from build123d import *

# Parameters (mm, degrees)
SKETCH1_W           = 60
SKETCH1_H           = 5
SKETCH1_W_2         = 50
SKETCH1_H_2         = 10
SKETCH1_W_3         = 5
BOSS_EXTRUDE1_DEPTH = 9
SKETCH1_3_W         = 50
SKETCH1_3_H         = 23
SKETCH1_3_W_2       = 65
SKETCH1_3_H_2       = 90
SKETCH1_3_R         = 1.5
SKETCH1_3_W_3       = 1.5
SKETCH1_3_H_3       = 74
BOSS_EXTRUDE2_DEPTH = 3
SKETCH2_R           = 1.5
BOSS_EXTRUDE3_DEPTH = 3
SKETCH3_R           = 4
CUT_EXTRUDE1_DEPTH  = 5
SKETCH3_3_R         = 1.5
CUT_EXTRUDE2_DEPTH  = 20
SKETCH4_W           = 70
SKETCH4_H           = 9
BOSS_EXTRUDE4_DEPTH = 3
SKETCH3_6_R         = 2.5
SKETCH3_6_R_2       = 1.5
CUT_EXTRUDE5_DEPTH  = 3


with BuildPart() as part:
    # Sketch1 → Boss-Extrude1 (new body)
    with BuildSketch(Plane(origin=(0, 0, 0), x_dir=(1, 0, 0), z_dir=(0, 1, 0))):
        Polygon((-30, -60), (-30, 40), (-30, 45), (-30, 65), (-35, 65), (-35, 25), (-35, -65), (-30, -65), align=None)
        with Locations((0, -62.5)):
            Rectangle(SKETCH1_W, SKETCH1_H)
        Polygon((30, 40), (30, -60), (30, -65), (35, -65), (35, 65), (30, 65), (30, 55), (30, 45), align=None)
        Polygon((-30, 65), (-30, 45), (-25, 45), (-25, 55), (25, 55), (25, 65), align=None)
        with Locations((0, 50)):
            Rectangle(SKETCH1_W_2, SKETCH1_H_2)
        with Locations((27.5, 60)):
            Rectangle(SKETCH1_W_3, SKETCH1_H_2)
        with Locations((27.5, 50)):
            Rectangle(SKETCH1_W_3, SKETCH1_H_2)
    extrude(amount=BOSS_EXTRUDE1_DEPTH)

    # Sketch1_3 → Boss-Extrude2 (add)
    # profile 1 of 2: a face of its own
    with BuildSketch(Plane(origin=(0, 0, 0), x_dir=(1, 0, 0), z_dir=(0, 1, 0))):
        Polygon((-30, 45), (-30, -60), (30, -60), (30, 45), (25, 45), (25, -23), (-25, -23), (-25, 45), align=None)
        with Locations((0, -43.5)):
            Rectangle(SKETCH1_3_W, SKETCH1_3_H, mode=Mode.SUBTRACT)
    # profile 2 of 2: a face of its own
    with BuildSketch(Plane(origin=(0, 0, 0), x_dir=(1, 0, 0), z_dir=(0, 1, 0))):
        with Locations((-67.5, -20)):
            Rectangle(SKETCH1_3_W_2, SKETCH1_3_H_2)
        with Locations(Location((-42.5, 22.5, 0), (0, 0, 270))):
            Circle(SKETCH1_3_R, mode=Mode.SUBTRACT)
        with Locations(Location((-57.5, -62.5, 0), (0, 0, 270))):
            Circle(SKETCH1_3_R, mode=Mode.SUBTRACT)
        with Locations(Location((-42.5, -62.5, 0), (0, 0, 270))):
            Circle(SKETCH1_3_R, mode=Mode.SUBTRACT)
        with Locations((-53, -20)):
            Rectangle(SKETCH1_3_W_3, SKETCH1_3_H_3, mode=Mode.SUBTRACT)
        with Locations(Location((-57.5, 22.5, 0), (0, 0, 270))):
            Circle(SKETCH1_3_R, mode=Mode.SUBTRACT)
        with Locations(Location((-77.5, 22.5, 0), (0, 0, 270))):
            Circle(SKETCH1_3_R, mode=Mode.SUBTRACT)
        with Locations(Location((-92.5, -62.5, 0), (0, 0, 270))):
            Circle(SKETCH1_3_R, mode=Mode.SUBTRACT)
        with Locations(Location((-77.5, -62.5, 0), (0, 0, 270))):
            Circle(SKETCH1_3_R, mode=Mode.SUBTRACT)
        with Locations((-88, -20)):
            Rectangle(SKETCH1_3_W_3, SKETCH1_3_H_3, mode=Mode.SUBTRACT)
        with Locations(Location((-92.5, 22.5, 0), (0, 0, 270))):
            Circle(SKETCH1_3_R, mode=Mode.SUBTRACT)
    extrude(amount=BOSS_EXTRUDE2_DEPTH)

    # Sketch2 → Boss-Extrude3 (add)
    with BuildSketch(Plane(origin=(0, 0, 0), x_dir=(1, 0, 0), z_dir=(0, 1, 0))):
        Polygon((35, -65), (-35, -65), (-100, -65), (-100, -70), (35, -70), align=None)
        with Locations(Location((30, -67.5, 0), (0, 0, 270))):
            Circle(SKETCH2_R, mode=Mode.SUBTRACT)
    extrude(amount=BOSS_EXTRUDE3_DEPTH)

    # Sketch3 → Cut-Extrude1 (cut)
    with BuildSketch(Plane(origin=(0, 9, 0), x_dir=(1, 0, 0), z_dir=(0, 1, 0))):
        with Locations(Location((-20, 58, 0), (0, 0, 270))):
            Circle(SKETCH3_R)
        with Locations(Location((20, 58, 0), (0, 0, 90))):
            Circle(SKETCH3_R)
    extrude(amount=-CUT_EXTRUDE1_DEPTH, mode=Mode.SUBTRACT)

    # Sketch3_3 → Cut-Extrude2 (cut)
    with BuildSketch(Plane(origin=(0, 9, 0), x_dir=(1, 0, 0), z_dir=(0, 1, 0))):
        with Locations(Location((30, 62.5, 0), (0, 0, 270))):
            Circle(SKETCH3_3_R)
    extrude(amount=-CUT_EXTRUDE2_DEPTH, mode=Mode.SUBTRACT)

    # Sketch4 → Boss-Extrude4 (add)
    with BuildSketch(Plane(origin=(0, 0, -65), x_dir=(-1, 0, 0), z_dir=(0, 0, -1))):
        with Locations((0, 4.5)):
            Rectangle(SKETCH4_W, SKETCH4_H)
    extrude(amount=BOSS_EXTRUDE4_DEPTH)

    # Sketch3_6 → Cut-Extrude5 (cut)
    with BuildSketch(Plane(origin=(0, 9, 0), x_dir=(1, 0, 0), z_dir=(0, 1, 0))):
        with Locations(Location((30, 62.5, 0), (0, 0, 270))):
            Circle(SKETCH3_6_R)
        with Locations(Location((30, 62.5, 0), (0, 0, 270))):
            Circle(SKETCH3_6_R_2, mode=Mode.SUBTRACT)
    extrude(amount=-CUT_EXTRUDE5_DEPTH, mode=Mode.SUBTRACT)


solid = part.part
Check sheet for the modelled part. Datum: model origin and axes. Units: mm. A direction names the side the tool comes from. Round coordinates to 2 decimals unless told otherwise and drop trailing zeros. Write each loop counter-clockwise with the first axis right and the second up, starting at its lowest first coordinate (ties: lowest second). Pieces come first, ordered by that corner, then holes. Notation, with made-up numbers: (-25.5, 52.25) - (-5.5, 52.25) arc R29 ccw to (-5.5, 73.25) - close; hole circle Ø5 at (33.5, 38). An arc over 180 degrees is marked (long way). Return JSON: item names as keys, results as strings.
Q1. Cross-section at D-D (z = -58). Record the boundary of the cut face in (x, y).
Returned:
{"outline": "(-35, 0) - (35, 0) - (35, 9) - (24, 9) - (24, 4) - (16, 4) - (16, 9) - (-16, 9) - (-16, 4) - (-24, 4) - (-24, 9) - (-35, 9) - close"}
Q2. Cross-section at A-A (x = 20). Record the boundary of the cut face in (y, z), then the cut area to 3 significant figures.
Returned:
{"outline": "(0, -68) - (9, -68) - (9, -62) - (4, -62) - (4, -54) - (9, -54) - (9, -45) - (0, -45) - close; (0, 23) - (3, 23) - (3, 32) - (0, 32) - close; (0, 55) - (3, 55) - (3, 60) - (9, 60) - (9, 65) - (3, 65) - (3, 70) - (0, 70) - close", "area": "269 mm²"}
Q3. Access from +Z, -Z, +X, -X, +Y, -Y to the whole of each face (thin tool, end or side, straight path). Record for faces 1 (the flat face through (-68, 1, -25)), 2 (the flat face through (20, 4, -58)), 3 (the flat face through (25, 1, 44)).
Returned:
{"face 1": "-Z, -X, +Y, -Y", "face 2": "+Y", "face 3": "+Y, -Y"}
Q4. Cross-section at B-B (z = -0.5). Record the boundary of the cut face in (x, y), then the cut area to 3 significant figures.
Returned:
{"outline": "(-100, 0) - (-88.75, 0) - (-88.75, 3) - (-100, 3) - close; (-87.25, 0) - (-53.75, 0) - (-53.75, 3) - (-87.25, 3) - close; (-52.25, 0) - (-25, 0) - (-25, 3) - (-30, 3) - (-30, 9) - (-35, 9) - (-35, 3) - (-52.25, 3) - close; (25, 0) - (35, 0) - (35, 9) - (30, 9) - (30, 3) - (25, 3) - close", "area": "306 mm²"}
Q5. Cross-section at C-C (z = -29). Record the boundary of the cut face in (x, y).
Returned:
{"outline": "(-35, 0) - (-25, 0) - (-25, 3) - (-30, 3) - (-30, 9) - (-35, 9) - close; (25, 0) - (35, 0) - (35, 9) - (30, 9) - (30, 3) - (25, 3) - close"}
Q6. Scan lines: L1, parallel to X at y = 1.5, z = -13; L2, parallel to X at y = 2.15, z = 62.5; L3, parallel to X at y = 7.9, z = -58. Record each from-to range of solid material in increasing order. Write a range as from..to.
Returned:
{"L1": "x = -100..-88.75, -87.25..-53.75, -52.25..-25, 25..35", "L2": "x = -100..-94, -91..-79, -76..-59, -56..-44, -41..35", "L3": "x = -35..-24, -16..16, 24..35"}
Q7. Depth check by flat-ended pin: P1, Ø8, axis at x = -71, z = 47.5, coming from the +Y side; P2, Ø2.5, axis at x = -68.5, y = 1, coming from the -Z side; P3, Ø4, axis at x = 30, z = -62.5, coming from the +Y side. Enter the tip coordinate at first touch or a pass-through.
Returned:
{"P1": "stops at y = 3", "P2": "stops at z = -25", "P3": "stops at y = 6"}
